from build123d import *

# Parameters (mm, degrees)
BOSS_EXTRU_1_DEPTH      = 75.755
ENL_V_MAT_EXTRU_1_DEPTH = 124.743757195
ENL_V_MAT_EXTRU_2_DEPTH = 164.948761341
ENL_V_MAT_EXTRU_3_DEPTH = 104.861599502
ESQUISSE7_R             = 4.1
ENL_V_MAT_EXTRU_8_DEPTH = 3


with BuildPart() as part:
    # Esquisse1 → Boss.-Extru.1 (new body)
    with BuildSketch(Plane(origin=(0, 18.275365242, 0), x_dir=(1, 0, 0), z_dir=(0, 1, 0))):
        Polygon((59.971997273, -14.940347022), (23.39332157, -4.940347022), (-35.499575309, -4.940347022), (-79.817340578, -9.940347022), (-79.817340578, -14.940347022), align=None)
    extrude(amount=BOSS_EXTRU_1_DEPTH)

    # Esquisse2 → Enlèv. mat.-Extru.1 (cut, through all)
    with BuildSketch(Plane.XY.offset(14.940347022)):
        Polygon((-79.817340578, 32.378172924), (-63.428173599, 69.489176305), (-61.786327919, 94.030365243), (-79.817340578, 94.030365243), align=None)
        Polygon((-10.515385045, 94.030365243), (-10.515385045, 83.030365243), (42.318963009, 83.030365243), (59.971997273, -17.829066981), (59.971997273, 94.030365243), align=None)
    extrude(amount=-ENL_V_MAT_EXTRU_1_DEPTH, mode=Mode.SUBTRACT)

    # Esquisse3 → Enlèv. mat.-Extru.2 (cut, through all)
    with BuildSketch(Plane.ZY.offset(79.817340578)):
        Polygon((4.940347022, 18.275365242), (9.940347022, 18.275365242), (4.940347022, 26.275365242), align=None)
        Polygon((4.940347022, 42.491079528), (4.940347022, 26.275365242), (9.940347022, 34.383222385), align=None)
        Polygon((4.940347022, 94.030365243), (4.940347022, 88.530365243), (9.940347022, 94.030365243), align=None)
        Polygon((4.940347022, 58.706793814), (4.940347022, 42.491079528), (9.940347022, 50.598936671), align=None)
        Polygon((4.940347022, 74.9225081), (4.940347022, 58.706793814), (9.940347022, 66.814650957), align=None)
        Polygon((4.940347022, 88.530365243), (4.940347022, 74.9225081), (9.940347022, 83.030365243), align=None)
    extrude(amount=-ENL_V_MAT_EXTRU_2_DEPTH, mode=Mode.SUBTRACT)

    # Esquisse4 → Enlèv. mat.-Extru.3 (cut, through all)
    with BuildSketch(Plane(origin=(0, 83.030365243, 0), x_dir=(1, 0, 0), z_dir=(0, 1, 0))):
        Polygon((23.39332157, -4.940347022), (-10.550727062, -4.940347022), (6.421297254, -9.940347022), align=None)
        Polygon((-10.550727062, -4.940347022), (-44.494775695, -4.940347022), (-27.522751379, -9.940347022), align=None)
        Polygon((-79.817340578, -4.940347022), (-61.934802033, -7.92281089), (-44.494775695, -4.940347022), align=None)
    extrude(amount=-ENL_V_MAT_EXTRU_3_DEPTH, mode=Mode.SUBTRACT)

    # Esquisse7 → Enlèv. mat.-Extru.8 (cut)
    with BuildSketch(Plane(origin=(0, 0, 14.940347022), x_dir=(-1, 0, 0), z_dir=(0, 0, -1))):
        with Locations((-41.152659422, 33.343031941)):
            Circle(ESQUISSE7_R)
    extrude(amount=ENL_V_MAT_EXTRU_8_DEPTH, mode=Mode.SUBTRACT)


solid = part.part
The listing builds one solid part. Answer for the finished solid, in the listing's coordinates (mm). A direction names the side the tool comes from. Round coordinates to 2 decimals unless told otherwise and drop trailing zeros. Order: outer loops, then holes, each group sorted by start corner. A loop starts at its lowest first (then second) coordinate and runs counter-clockwise, first axis right, second up. Notation, with made-up numbers: (67.5, 74) -> (101.5, 74) arc R11 ccw to (101.5, 93) -> close; hole circle Ø4 at (12.5, -29.75). An arc over 180 degrees is marked (long way). Put each result on its own line as item: value.
Q1. Each of these flat-tipped pins is pushed along its axis until it touches: P1, Ø9.5, axis at x = 41.15, y = 33.34, coming from the -Z side; P2, Ø3, axis at y = 84.5, z = 8.5, coming from the -X side; P3, Ø3, axis at y = 90.5, z = 12, coming from the +X side. Where does it stop, or does it pass through?
Results list:
P1: z = 8.54
P2: x = -62.49
P3: x = -10.52
Q2. Determine the mould class of faces 1 (the flat face through (-33.26, 58.82, 8.25)), 2 (the flat face through (-54.933, 74.79, 7.133)), 3 (the flat face through (-46.902, 64.076, 8.251)) for opening direction X: pulls with the +X half, pulls with the -X half, needs draft (parallel to the pull), parting line crosses it, or undercut.
Results list:
face 1: undercut
face 2: pulls with the -X half
face 3: needs draft
Q3. Section D-D, the plane y = 86.5 is taken. Write down the section's boundary in (x, z), and give its area (3 significant figures).
Results list:
outline: (-62.29, 7.96) -> (-51.86, 6.79) -> (-10.52, 6.79) -> (-10.52, 14.94) -> (-62.29, 14.94) -> close
area: 416 mm^2
Q4. Section B-B, the plane y = 65.5 is taken. Write down the section's boundary in (x, z), and give its area (3 significant figures).
Results list:
outline: (-65.19, 9.13) -> (-30.27, 9.13) -> (-27.52, 9.94) -> (-24.77, 9.13) -> (3.67, 9.13) -> (6.42, 9.94) -> (9.17, 9.13) -> (38.72, 9.13) -> (45.39, 10.95) -> (45.39, 14.94) -> (-65.19, 14.94) -> close
area: 632 mm^2
Q5. Which of the six approach directions +Z, -Z, +X, -X, +Y, -Y give full straight-line access (tool end or side, diameter ignored) to faces 4 (the flat face through (12.9, 75.04, 8.03)), 5 (the flat face through (-21.04, 75.04, 8.03)), 6 (the flat face through (-10.79, 47.39, 7.96))?
Results list:
face 4: -Z, +Y, -Y
face 5: -Z, -Y
face 6: -Z, +X, -X
Q6. Section C-C, the plane x = -30 is taken. Write down the section's boundary in (y, z), and give its area (3 significant figures).
Results list:
outline: (18.28, 9.94) -> (19.44, 9.21) -> (33.2, 9.21) -> (34.38, 9.94) -> (35.57, 9.21) -> (49.42, 9.21) -> (50.6, 9.94) -> (51.78, 9.21) -> (65.63, 9.21) -> (66.81, 9.94) -> (68, 9.21) -> (81.85, 9.21) -> (83.03, 9.94) -> (88.53, 4.94) -> (94.03, 9.94) -> (94.03, 14.94) -> (18.28, 14.94) -> close
area: 450 mm^2
Q7. Consider line 1 along Y through (x, z) = (-23, 8.75); line 2 along Y through (x, z) = (-45, 9.75); line 3 along Z through (x, y) = (-37.5, 67). Determine where each line is inside the solid, lowest interval first.
Results list:
line 1: 20.18 to 32.45, 36.31 to 48.67, 52.53 to 64.88, 68.74 to 81.1, 84.34 to 92.72
line 2: 18.58 to 34.07, 34.69 to 50.29, 50.91 to 66.51, 67.12 to 82.72, 83.24 to 93.82
line 3: 9.83 to 14.94
Q8. Section A-A, the plane x = 4 is taken. Write down the section's boundary in (y, z), and give its area (3 significant figures).
Results list:
outline: (18.28, 9.94) -> (19.42, 9.23) -> (33.23, 9.23) -> (34.38, 9.94) -> (35.54, 9.23) -> (49.44, 9.23) -> (50.6, 9.94) -> (51.76, 9.23) -> (65.66, 9.23) -> (66.81, 9.94) -> (67.97, 9.23) -> (81.87, 9.23) -> (83.03, 9.94) -> (83.03, 14.94) -> (18.28, 14.94) -> close
area: 367 mm^2
